Source: CAD feature listing. Evaluate the final solid. Frame: model axes, mm. Give positions to 0.01 mm unless a question says otherwise; leave off trailing zeros. Loops run counter-clockwise (first coordinate to the right, second up) from the corner with the lowest first, then second, coordinate; pieces in that order, holes last. Notation, with made-up numbers: (-28.5, 1.25) -> (-7.5, 1.25) arc R19 ccw to (-7.5, 22.25) -> close; hole circle Ø11 at (-29.5, 76.5). An arc over 180 degrees is marked (long way). Answer as a JSON object with one key per item and string values. Group by question number.
from build123d import *

# Parameters (mm, degrees)
F1_DEPTH = 52
F2_R     = 11
F3_DEPTH = 38
F6_R     = 25


with BuildPart() as f1:
    # F0 (on Top) → F1 (new body)
    with BuildSketch(Plane.XY):
        with BuildLine():
            Line((182, 38), (62.329768, 38))
            ThreePointArc((62.329768, 38), (-19.734829, 70.281836), (-73, 0))
            Line((-73, 0), (182, 0))
            Line((182, 0), (182, 38))
        make_face()
    extrude(amount=F1_DEPTH)

    # F2 (on face) → F3 (cut)
    with BuildSketch(Plane.XZ):
        with Locations((109, 26)):
            Circle(F2_R)
        with Locations((157, 26)):
            Circle(F2_R)
    extrude(amount=-F3_DEPTH, mode=Mode.SUBTRACT)

    # F4 (on face) → F5 (revolve, cut)
    with BuildSketch(Plane.XZ):
        Polygon((0, 0), (0, 52), (-60, 52), (-42, 0), align=None)
    revolve(axis=Axis((0, 0, 26), (0, 0, 1)), mode=Mode.SUBTRACT)

    # F6
    f6_edges = [f1.edges().sort_by_distance(p)[0] for p in [
        (182, 19, 52),
        (182, 19, 0),
    ]]
    fillet(f6_edges, radius=F6_R)


solid = f1.part
(1) Section query C-C on y = 6. State how many separate pieces and enclosed holes the cut face has, plus the area to 3 significant figures.
(2) Material intervals for line 1 (Z direction, x = 157, y = 28); line 2 (X direction, y = 13.5, z = 32.5); line 3 (X direction, y = 23.5, z = 41), sorted ascending. Write a range as from..to.
(3) Section query A-A on x = 109. Return the cut outline in (y, z), plus the area to 3 significant figures.
(4) Section query B-B on z = 33. Return the cut outline in (x, y).
(5) First-contact query: pin 1 (5 mm diameter, centred on x = -11, z = 43, fed in from +Y); pin 2 (2 mm diameter, centred on x = 122, z = 37.5, fed in from +Y); pin 3 (13 mm diameter, centred on x = 157, z = 26, fed in from -Y); pin 4 (1.5 mm diameter, centred on y = 62.5, z = 11.5, fed in from +X). Flat tips, straight axial feed; report the tip coordinate or a pass-through.
(6) Section query D-D on z = 19.5. Return the cut outline in (x, y).
(7) Mould query, pull axis X, two halves, no side actions, for faces 1 (the face through (123, 38, 26)), 2 (the face through (-18.455, 70.629, 25.636)), 3 (the face through (1.075, 48.862, 19.858)), 4 (the face through (174.871, 19.266, 44.482)). Classes: pulls with the +X half, pulls with the -X half, needs draft (parallel to the pull), parting line crosses it, or undercut.
Result:
{
 "1": {"separate pieces": "2", "enclosed holes": "2", "area": "6,950 mm²"},
 "2": {"line 1": "0..15, 37..52", "line 2": "-71.74..-51.51, 51.51..100.13, 117.87..148.13, 165.87..181.39", "line 3": "-69.11..-51.04, 51.04..177.71"},
 "3": {"outline": "(0, 0) -> (38, 0) -> (38, 15) -> (0, 15) -> close; (0, 37) -> (38, 37) -> (38, 52) -> (0, 52) -> close", "area": "1,140 mm²"},
 "4": {"outline": "(-73, 0) -> (-53.42, 0) arc R53.42 cw to (53.42, 0) -> (100.51, 0) -> (100.51, 38) -> (62.33, 38) arc R73 ccw to start; (117.49, 0) -> (148.51, 0) -> (148.51, 38) -> (117.49, 38) -> close; (165.49, 0) -> (181.27, 0) -> (181.27, 38) -> (165.49, 38) -> close"},
 "5": {"pin 1": "y = 72.5", "pin 2": "y = 38", "pin 3": "through", "pin 4": "x = 38.94"},
 "6": {"outline": "(-73, 0) -> (-48.75, 0) arc R48.75 cw to (48.75, 0) -> (100.13, 0) -> (100.13, 38) -> (62.33, 38) arc R73 ccw to start; (117.87, 0) -> (148.13, 0) -> (148.13, 38) -> (117.87, 38) -> close; (165.87, 0) -> (181.39, 0) -> (181.39, 38) -> (165.87, 38) -> close"},
 "7": {"face 1": "needs draft", "face 2": "parting line crosses it", "face 3": "undercut", "face 4": "pulls with the +X half"}
}
